The model under review builds one solid part; all positions refer to its coordinate system, in mm. Face numbers are marked on the shaded views. A direction names the side the tool comes from. Give positions to 0.01 mm unless a question says otherwise; leave off trailing zeros. Loops run counter-clockwise (first coordinate to the right, second up) from the corner with the lowest first, then second, coordinate; pieces in that order, holes last. Notation, with made-up numbers: M -14.5,82.5 L 27.5,82.5 A11 ccw 27.5,98.5 Z; hole C 16,75.25 d10. An arc over 180 degrees is marked long. Return JSON: item names as keys, results as strings.
```python
from build123d import *

# Parameters (mm, degrees)
SKETCH1_W           = 50
SKETCH1_H           = 30
BOSS_EXTRUDE1_DEPTH = 30
SKETCH3_R           = 5
CUT_EXTRUDE1_DEPTH  = 40
SKETCH4_W           = 1.254965376
SKETCH4_H           = 1
CUT_EXTRUDE2_DEPTH  = 61.207972894
SKETCH5_R           = 2.5
SKETCH5_R_2         = 2.597055459
CUT_EXTRUDE3_DEPTH  = 18
BOSS_EXTRUDE2_START = 5
SKETCH6_R           = 3.75
SKETCH6_R_2         = 2.597055459
BOSS_EXTRUDE2_DEPTH = 5
SKETCH7_R           = 2.5
CUT_EXTRUDE4_DEPTH  = 5
SKETCH8_R           = 3.5
SKETCH8_R_2         = 2.5
BOSS_EXTRUDE3_DEPTH = 10
SKETCH9_R           = 1
CUT_EXTRUDE5_DEPTH  = 56
FILLET1_R           = 10


with BuildPart() as part:
    # Sketch1 → Boss-Extrude1 (new body)
    with BuildSketch(Plane(origin=(0, 0, 0), x_dir=(0, 0, -1), z_dir=(1, 0, 0))):
        Rectangle(SKETCH1_W, SKETCH1_H)
    extrude(amount=BOSS_EXTRUDE1_DEPTH)

    # Sketch3 → Cut-Extrude1 (cut)
    with BuildSketch(Plane(origin=(0, 0, -25), x_dir=(-1, 0, 0), z_dir=(0, 0, -1))):
        with Locations((-15, 0)):
            Circle(SKETCH3_R)
    extrude(amount=-CUT_EXTRUDE1_DEPTH, mode=Mode.SUBTRACT)

    # Sketch4 → Cut-Extrude2 (cut, through all)
    with BuildSketch(Plane(origin=(0, 0, -25), x_dir=(-1, 0, 0), z_dir=(0, 0, -1))):
        with Locations((-29.372517312, 6.5)):
            Rectangle(SKETCH4_W, SKETCH4_H)
        with Locations((-29.372517312, -6.5)):
            Rectangle(SKETCH4_W, SKETCH4_H)
        with Locations((-0.627482688, -6.5)):
            Rectangle(SKETCH4_W, SKETCH4_H)
        with Locations((-0.627482688, 6.5)):
            Rectangle(SKETCH4_W, SKETCH4_H)
    extrude(amount=-CUT_EXTRUDE2_DEPTH, mode=Mode.SUBTRACT)

    # Sketch5 → Cut-Extrude3 (cut)
    with BuildSketch(Plane(origin=(0, 15, 0), x_dir=(1, 0, 0), z_dir=(0, 1, 0))):
        with Locations(Location((15, 20, 0), (0, 0, 270))):
            Circle(SKETCH5_R)
        with Locations(Location((15, -20, 0), (0, 0, 270))):
            Circle(SKETCH5_R_2)
    extrude(amount=-CUT_EXTRUDE3_DEPTH, mode=Mode.SUBTRACT)

    # Sketch6 → Boss-Extrude2 (add)
    # profile 1 of 2: a face of its own
    with BuildSketch(Plane(origin=(0, 15, 0), x_dir=(1, 0, 0), z_dir=(0, 1, 0)).offset(BOSS_EXTRUDE2_START)):
        with Locations(Location((15, -20, 0), (0, 0, 90))):
            Circle(SKETCH6_R)
        with Locations(Location((15, -20, 0), (0, 0, 270))):
            Circle(SKETCH6_R_2, mode=Mode.SUBTRACT)
    # profile 2 of 2: a face of its own
    with BuildSketch(Plane(origin=(0, 15, 0), x_dir=(1, 0, 0), z_dir=(0, 1, 0)).offset(BOSS_EXTRUDE2_START)):
        with Locations(Location((15, 20, 0), (0, 0, 90))):
            Circle(SKETCH6_R)
        with Locations(Location((15, 20, 0), (0, 0, 270))):
            Circle(SKETCH6_R_2, mode=Mode.SUBTRACT)
    extrude(amount=-BOSS_EXTRUDE2_DEPTH)

    # Sketch7 → Cut-Extrude4 (cut)
    with BuildSketch(Plane(origin=(0, 0, 15), x_dir=(-1, 0, 0), z_dir=(0, 0, -1))):
        with Locations((-15, 0)):
            Circle(SKETCH7_R)
    extrude(amount=-CUT_EXTRUDE4_DEPTH, mode=Mode.SUBTRACT)

    # Sketch8 → Boss-Extrude3 (add)
    with BuildSketch(Plane.XY.offset(25)):
        with Locations(Location((14.885614907, 0, 0), (0, 0, 180))):
            Circle(SKETCH8_R)
        with Locations((14.885614907, 0)):
            Circle(SKETCH8_R_2, mode=Mode.SUBTRACT)
    extrude(amount=BOSS_EXTRUDE3_DEPTH)

    # Sketch9 → Cut-Extrude5 (cut, through all)
    with BuildSketch(Plane(origin=(0, 15, 0), x_dir=(1, 0, 0), z_dir=(0, 1, 0))):
        with Locations(Location((14.885614907, -32.5, 0), (0, 0, 270))):
            Circle(SKETCH9_R)
    extrude(amount=-CUT_EXTRUDE5_DEPTH, mode=Mode.SUBTRACT)

    # Fillet1
    # the kernel refuses this fillet: 10 mm, written as the material it takes off along each edge
    with BuildSketch(Plane(origin=(30, -15, 49.494897428), x_dir=(-1, 0, 0), z_dir=(0, 0, -1)), Plane(origin=(30, 15, -49.494897428), x_dir=(-1, 0, 0), z_dir=(0, 0, 1))) as fillet1_piece_1:
        with BuildLine():
            CenterArc((9.797958971, 10), FILLET1_R, 191.536959033, 78.463040967)
            Line((0, 8), (-0.195959179, 7.96))
            ThreePointArc((-0.195959179, 7.96), (-0.2, 4), (-0.2, 0))
            Line((-0.2, 0), (0, -0.2))
            Line((0, -0.2), (9.797958971, -0.2))
            Line((9.797958971, -0.2), (9.797958971, 0))
        make_face()
    extrude(amount=98.989794856, mode=Mode.SUBTRACT)
    with BuildSketch(Plane(origin=(0, -15, 49.494897428), x_dir=(1, 0, 0), z_dir=(0, 0, -1))) as fillet1_piece_2:
        with BuildLine():
            CenterArc((9.797958971, -10), FILLET1_R, 90, 78.463040967)
            Line((0, -8), (-0.195959179, -7.96))
            ThreePointArc((-0.195959179, -7.96), (-0.2, -4), (-0.2, 0))
            Line((-0.2, 0), (0, 0.2))
            Line((0, 0.2), (9.797958971, 0.2))
            Line((9.797958971, 0.2), (9.797958971, 0))
        make_face()
    extrude(amount=98.989794856, mode=Mode.SUBTRACT)
    with BuildSketch(Plane(origin=(0, 15, -49.494897428), x_dir=(0, -1, 0), z_dir=(0, 0, 1))) as fillet1_piece_3:
        with BuildLine():
            CenterArc((10, 9.797958971), FILLET1_R, 180, 78.463040967)
            Line((0, 9.797958971), (-0.2, 9.797958971))
            Line((-0.2, 9.797958971), (-0.2, 0))
            Line((-0.2, 0), (0, -0.2))
            ThreePointArc((0, -0.2), (4, -0.2), (7.96, -0.195959179))
            Line((7.96, -0.195959179), (8, 0))
        make_face()
    extrude(amount=98.989794856, mode=Mode.SUBTRACT)


solid = part.part
```
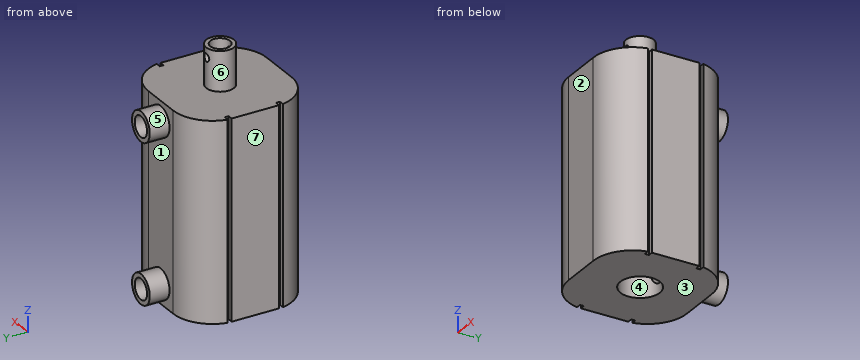
1) Wall thickness on L1, parallel to Z at x = 15, y = 12.75; L2, parallel to Z at x = 2.5, y = -7; L3, parallel to Z at x = 16, y = 16: over which ranges is each line inside the solid? List them lowest first. Write a range as from..to.
From the geometry:
{"L1": "-25..-22.5, -17.5..17.4, 22.6..25", "L2": "-25..25", "L3": "-23.61..-22.4, -17.6..-16.39, 16.39..17.6, 22.4..23.61"}
2) Insertion check: pin 1 (8 mm diameter, centred on x = 15, y = 0, fed in from -Z); pin 2 (2.5 mm diameter, centred on x = 14.89, z = 32.5, fed in from -Y); pin 3 (3 mm diameter, centred on x = 6, z = 1.5, fed in from -Y). Each pin has a flat end and moves straight along its axis. Give the tip position at first contact, or say it passes through.
From the geometry:
{"pin 1": "z = 15", "pin 2": "y = -3.5", "pin 3": "y = -14.73"}
3) Consider section A-A on z = 5.5. Write out the cut boundary in (x, y), then the cut area to 3 significant figures.
From the geometry:
{"outline": "M 0,-7 A10 ccw 9.8,-15 L 20.2,-15 A10 ccw 30,-7 L 28.75,-7 L 28.75,-6 L 30,-6 L 30,6 L 28.75,6 L 28.75,7 L 30,7 A10 ccw 20.2,15 L 9.8,15 A10 ccw 0,7 L 1.25,7 L 1.25,6 L 0,6 L 0,-6 L 1.25,-6 L 1.25,-7 Z; hole C 15,0 d10", "area": "738 mm²"}
4) Consider section B-B on y = 0. Write out the cut boundary in (x, z), then the cut area to 3 significant figures.
From the geometry:
{"outline": "M 0,-25 L 10,-25 L 10,15 L 12.5,15 L 12.5,19.3 A2.6 cw long 17.5,19.3 L 17.5,15 L 20,15 L 20,-25 L 30,-25 L 30,25 L 18.39,25 L 18.39,35 L 17.39,35 L 17.39,25 L 12.39,25 L 12.39,35 L 11.39,35 L 11.39,25 L 0,25 Z", "area": "1,080 mm²"}
5) The part is to be moulded in two halves that separate along Z. For the marked faces 1, 2 and 3, say which applies: released by +Z, released by -Z, zero draft, split by the parting line, or undercut.
From the geometry:
{"face 1": "undercut", "face 2": "zero draft", "face 3": "released by -Z"}
6) Consider section C-C on y = 17. Write out the cut boundary in (x, z).
From the geometry:
{"outline": "C 15,-20 d7.5; C 15,20 d7.5; hole C 15,-20 d5.19; hole C 15,20 d5.19"}
7) Tool access review of the marked faces 4, 5, 6 and 7: name each direction out of +Z, -Z, +X, -X, +Y, -Y from which nothing blocks a thin tool from reaching the whole face with its end or side.
From the geometry:
{"face 4": "-Z", "face 5": "+Y", "face 6": "+Z", "face 7": "+Z, -Z, -X, +Y, -Y"}
